For this review, take the finished solid that the model builds, in its own axes (mm). Face numbers are marked on the shaded views. A direction names the side the tool comes from. Round coordinates to 2 decimals unless told otherwise and drop trailing zeros. Order: outer loops, then holes, each group sorted by start corner. A loop starts at its lowest first (then second) coordinate and runs counter-clockwise, first axis right, second up. Notation, with made-up numbers: (60.25, 63) -> (89.25, 63) arc R27 ccw to (89.25, 81) -> close; hole circle Ø4 at (81, 10.5). An arc over 180 degrees is marked (long way). Answer in a Markdown table with one row per item.
```python
from build123d import *

# Parameters (mm, degrees)
EXTRUDE_1_DEPTH     = 5
SKETCH_2_R          = 1.6
SKETCH_2_W          = 40
SKETCH_2_H          = 40
CUT_EXTRUDE_1_DEPTH = 86
FILLET_1_R          = 10


with BuildPart() as part:
    # 草图1 → 凸台-拉伸1 (new body)
    with BuildSketch(Plane.XY):
        with BuildLine():
            Line((5, 0), (55, 0))
            ThreePointArc((55, 0), (58.535533906, 1.464466094), (60, 5))
            Line((60, 5), (60, 55))
            ThreePointArc((60, 55), (58.535533906, 58.535533906), (55, 60))
            Line((55, 60), (5, 60))
            ThreePointArc((5, 60), (1.464466094, 58.535533906), (0, 55))
            Line((0, 55), (0, 5))
            ThreePointArc((0, 5), (1.464466094, 1.464466094), (5, 0))
        make_face()
    extrude(amount=EXTRUDE_1_DEPTH)

    # 草图2 → 切除-拉伸1 (cut, through all)
    with BuildSketch(Plane.XY.offset(5)):
        with Locations((5, 55)):
            Circle(SKETCH_2_R)
        with Locations((30, 55)):
            Circle(SKETCH_2_R)
        with Locations((55, 55)):
            Circle(SKETCH_2_R)
        with Locations((55, 30)):
            Circle(SKETCH_2_R)
        with Locations((30, 5)):
            Circle(SKETCH_2_R)
        with Locations((55, 5)):
            Circle(SKETCH_2_R)
        with Locations((5, 30)):
            Circle(SKETCH_2_R)
        with Locations((5, 5)):
            Circle(SKETCH_2_R)
        with Locations((30, 30)):
            Rectangle(SKETCH_2_W, SKETCH_2_H)
    extrude(amount=-CUT_EXTRUDE_1_DEPTH, mode=Mode.SUBTRACT)

    # 圆角1
    fillet_1_edges = [part.edges().sort_by_distance(p)[0] for p in [
        (10, 10, 2.5),
        (10, 50, 2.5),
        (50, 50, 2.5),
        (50, 10, 2.5),
    ]]
    fillet(fillet_1_edges, radius=FILLET_1_R)


solid = part.part
```
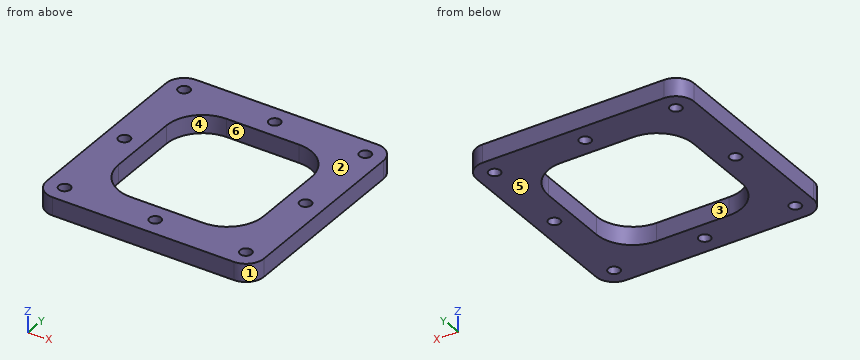
Q1. Take a section at C-C, the plane z = 2.4. Give the number of separate pieces and of enclosed holes in the cut face, then the cut area to 3 significant figures.
Answer key:
| item | result |
|---|---|
| separate pieces | 1 |
| enclosed holes | 9 |
| area | 2,000 mm^2 |
Q2. Clearance check with a flat-ended pin moving along its axis: pin 1 Ø3 at (x, y) = (5, 55) entering from +Z. State where the tip first meets the part, or that it passes through.
Answer key:
| item | result |
|---|---|
| pin 1 | passes through |
Q3. To check wall thickness, follow probe 1 along X at (y, z) = (26.5, 2.95); probe 2 along Y at (x, z) = (30, 0.45). State the ranges of each line that lie inside material, in increasing order.
Answer key:
| item | result |
|---|---|
| probe 1 | x = 0 to 10, 50 to 60 |
| probe 2 | y = 0 to 3.4, 6.6 to 10, 50 to 53.4, 56.6 to 60 |
Q4. Take a section at B-B, the plane x = 46. Write out the cut boundary in (y, z), then the cut area to 3 significant figures.
Answer key:
| item | result |
|---|---|
| outline | (0, 0) -> (12, 0) -> (12, 5) -> (0, 5) -> close; (48, 0) -> (60, 0) -> (60, 5) -> (48, 5) -> close |
| area | 120 mm^2 |
Q5. The part is to be moulded in two halves that separate along X. For the marked faces 1, 2, 3 and 4, say which applies: +X half, -X half, draft (parallel to the pull), parting line (faces both ways), or undercut.
Answer key:
| item | result |
|---|---|
| face 1 | +X half |
| face 2 | draft |
| face 3 | undercut |
| face 4 | undercut |
Q6. Tool access review of the marked faces 5 and 6: name each direction out of +Z, -Z, +X, -X, +Y, -Y from which nothing blocks a thin tool from reaching the whole face with its end or side.
Answer key:
| item | result |
|---|---|
| face 5 | -Z, +X, -X, +Y, -Y |
| face 6 | +Z, -Z |
Q7. Take a section at A-A, the plane x = 30. Write out the cut boundary in (y, z).
Answer key:
| item | result |
|---|---|
| outline | (0, 0) -> (3.4, 0) -> (3.4, 5) -> (0, 5) -> close; (6.6, 0) -> (10, 0) -> (10, 5) -> (6.6, 5) -> close; (50, 0) -> (53.4, 0) -> (53.4, 5) -> (50, 5) -> close; (56.6, 0) -> (60, 0) -> (60, 5) -> (56.6, 5) -> close |
